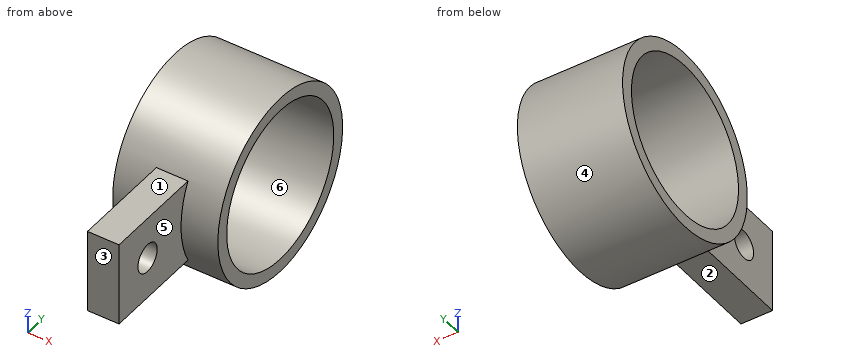
from build123d import *

# Parameters (mm, degrees)
COLLAR_SKETCH_W         = 20
COLLAR_SKETCH_H         = 2.48
TAB_SKETCH_W            = 6
TAB_SKETCH_H            = 26.896697694
TAB_DEPTH               = 8
TUBE_CLEARANCE_SKETCH_W = 8
TUBE_CLEARANCE_SKETCH_H = 15.02
PIN_HOLE_SKETCH_R       = 2.7
PIN_HOLE_DEPTH          = 6


with BuildPart() as part:
    # Collar Sketch → Collar (revolve)
    with BuildSketch(Plane.XY, mode=Mode.PRIVATE) as collar_sk:
        with Locations((242.635235803, 16.26)):
            Rectangle(COLLAR_SKETCH_W, COLLAR_SKETCH_H)
    revolve(collar_sk.sketch.rotate(Axis((-3000, 0, 0), (1, 0, 0)), 90), axis=Axis((-3000, 0, 0), (1, 0, 0)))

    # Tab Sketch → Tab (add, symmetric)
    with BuildSketch(Plane.XY):
        with Locations((242.635235803, -21.448348847)):
            Rectangle(TAB_SKETCH_W, TAB_SKETCH_H)
    extrude(amount=TAB_DEPTH, both=True)

    # Tube Clearance Sketch → Tube Clearance (revolve, cut)
    with BuildSketch(Plane.XY):
        with Locations((242.635235803, 7.51)):
            Rectangle(TUBE_CLEARANCE_SKETCH_W, TUBE_CLEARANCE_SKETCH_H)
    revolve(axis=Axis((-3000, 0, 0), (1, 0, 0)), mode=Mode.SUBTRACT)

    # Pin Hole Sketch → Pin Hole (cut)
    with BuildSketch(Plane(origin=(239.635235803, 0, 0), x_dir=(0, 0, -1), z_dir=(1, 0, 0))):
        with Locations((0, -26.896697694)):
            Circle(PIN_HOLE_SKETCH_R)
    extrude(amount=PIN_HOLE_DEPTH, mode=Mode.SUBTRACT)


solid = part.part
Verification items for the finished model (mm, model axes). Face numbers are marked on the shaded views. A direction names the side the tool comes from. Give positions to 0.01 mm unless a question says otherwise; leave off trailing zeros. Loops run counter-clockwise (first coordinate to the right, second up) from the corner with the lowest first, then second, coordinate; pieces in that order, holes last.
1) Draft check along Y on the marked faces 3, 4, 5 and 6. Enter one of: pulls with the +Y half, pulls with the -Y half, needs draft (parallel to the pull), parting line crosses it, or undercut.
2) Set-up check for the marked faces 1 and 2: record each of +Z, -Z, +X, -X, +Y, -Y from which the full face is reachable in a straight line by a thin tool's end or side.
3) Sectioned sample at C-C, the plane x = 242. Enter the section's corners in (y, z), then the cut area to 3 significant figures.
4) Sectioned sample at B-B, the plane y = 0. Enter the section's corners in (x, z).
5) Thickness scan on line 1 along Y through (x, z) = (242.55, 0); line 2 along X through (y, z) = (-25, 2.5); line 3 along Z through (x, y) = (245.25, -1). Record the ranges inside material, lowest first.
6) Sectioned sample at A-A, the plane z = 0. Enter the section's corners in (x, y), then the cut area to 3 significant figures.
7) Depth check by flat-ended pin: pin 1 Ø4 at (x, z) = (249.5, -3.5) entering from -Y; pin 2 Ø17.5 at (y, z) = (-29.5, -3.5) entering from +X; pin 3 Ø6.5 at (x, y) = (242.5, -28.5) entering from +Z; pin 4 Ø1 at (y, z) = (-15, 10.5) entering from -X. Enter the tip coordinate at first touch or a pass-through.
8) Sectioned sample at D-D, the plane z = 4. Enter the section's corners in (x, y), then the cut area to 3 significant figures.
Answers:
1. face 3: pulls with the -Y half
1. face 4: parting line crosses it
1. face 5: needs draft
1. face 6: undercut
2. face 1: +Z, +X, -X, -Y
2. face 2: -Z, +X, -X, -Y
3. outline: (-34.9, -8) - (-15.56, -8) arc R17.5 ccw (long way) to (-15.56, 8) - (-34.9, 8) - close; hole circle Ø5.4 at (-26.9, 0); hole circle Ø30.04 at (0, 0)
3. area: 519 mm2
4. outline: (232.64, -17.5) - (252.64, -17.5) - (252.64, -15.02) - (232.64, -15.02) - close; (232.64, 15.02) - (252.64, 15.02) - (252.64, 17.5) - (232.64, 17.5) - close
5. line 1: y = -34.9 to -29.6, -24.2 to -15.02, 15.02 to 17.5
5. line 2: x = 239.64 to 245.64
5. line 3: z = -17.47 to -14.99, 14.99 to 17.47
6. outline: (232.64, -17.5) - (239.64, -17.5) - (239.64, -24.2) - (245.64, -24.2) - (245.64, -17.5) - (252.64, -17.5) - (252.64, -15.02) - (232.64, -15.02) - close; (232.64, 15.02) - (252.64, 15.02) - (252.64, 17.5) - (232.64, 17.5) - close; (239.64, -34.9) - (245.64, -34.9) - (245.64, -29.6) - (239.64, -29.6) - close
6. area: 171 mm2
7. pin 1: stops at y = -17.44
7. pin 2: stops at x = 245.64
7. pin 3: stops at z = 8
7. pin 4: passes through
8. outline: (232.64, -17.04) - (239.64, -17.04) - (239.64, -34.9) - (245.64, -34.9) - (245.64, -17.04) - (252.64, -17.04) - (252.64, -14.48) - (232.64, -14.48) - close; (232.64, 14.48) - (252.64, 14.48) - (252.64, 17.04) - (232.64, 17.04) - close
8. area: 210 mm2
